Here's how the part is built. I have some questions about the finished solid (model axes, mm). Face numbers are marked on the shaded views. A direction names the side the tool comes from. Coordinates: 2 decimals unless noted, no trailing zeros. Order: outer loops, then holes, each group sorted by start corner. A loop starts at its lowest first (then second) coordinate and runs counter-clockwise, first axis right, second up.
Autodesk Inventor part; units mm, degrees
ref_plane "YZ Plane" through (0, 0, 0) normal (1, 0, 0) x (0, 1, 0)
ref_plane "XZ Plane" through (0, 0, 0) normal (0, 1, 0) x (-1, 0, 0)
ref_plane "XY Plane" through (0, 0, 0) normal (0, 0, 1) x (1, 0, 0)
sketch "Sketch1" plane through (0, 0, 0) normal (0, 0, 1) x (1, 0, 0)
  circle A0 centre (0, 0) radius 5
  dimension "d0" = 10
extrude "Extrusion1" add sketch "Sketch1" along normal blind 3
sketch "Sketch2" plane through (0, 0, 3) normal (0, 0, 1) x (1, 0, 0)
  circle A0 centre (0, 0) radius 5
  line L0 (-5.1933, 1) -> (5.1933, 1)
  line L1 (5.1933, 1) -> (5.1933, -1)
  line L2 (5.1933, -1) -> (-5.1933, -1)
  line L3 (-5.1933, -1) -> (-5.1933, 1)
  line L4 (-5.1933, 1) -> (5.1933, -1) construction
  line L5 (5.1933, 1) -> (-5.1933, -1) construction
  point P0 (-4.899, -1)
  point P1 (4.899, -1)
  point P2 (4.899, 1)
  point P3 (-4.899, 1)
  dimension "d3" = 2
  dimension "d4" = 79.101
extrude "Extrusion2" cut sketch "Sketch2" against normal blind 1 contours A0 L2 L0
fillet "Fillet1" radius 1 2 edges at (0, 5, 3) (0, -5, 3)
sketch "Sketch3" plane through (0, 0, 0) normal (0, 0, -1) x (-1, 0, 0)
  circle A0 centre (0, 0) radius 5
  circle A1 centre (0, 0) radius 3.25
  dimension "d8" = 6.5
extrude "Extrusion3" add sketch "Sketch3" along normal blind 16 contours A1
sketch "Sketch4" plane through (0, 0, -16) normal (0, 0, -1) x (-1, 0, 0)
  circle A0 centre (0, 0) radius 3.25
hole "Hole1" at (0, 0, -16) direction (0, 0, 1) diameter 3.242 depth 8 tip angle 118
properties part number "17B - Crosshead Pin2" material "Steel AISI 1020 107 HR"
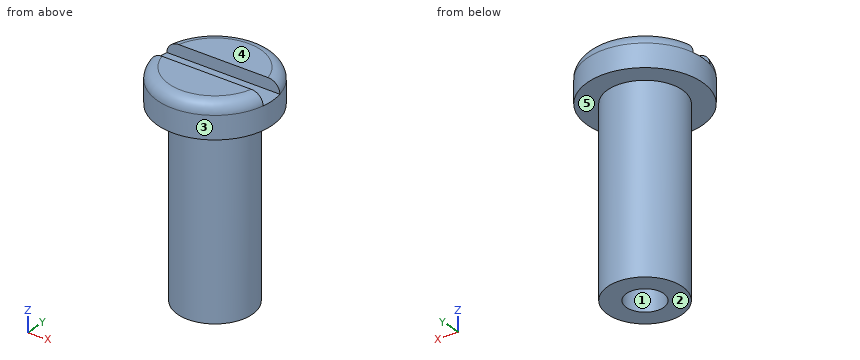
Q1. If we section it at C-C on z = -4: Write out the boundary of the cut face in (x, y), then the cut area to 3 significant figures.
Q2. For the marked faces 4 and 5, which set-ups out of +Z, -Z, +X, -X, +Y, -Y let a thin tool reach every point of the face, with its end or its side?
Q3. If we section it at A-A on z = -11: Write out the boundary of the cut face in (x, y).
Q4. I need wall thicknesses on L1, parallel to Y at x = 0, z = -12; L2, parallel to Z at x = -2, y = -0.5; L3, parallel to Z at x = -3, y = 2.25. Which ranges of each line are inside material? Lowest first, please.
Q5. We'd pull the mould along Y, two halves only. Please class the marked faces 1, 2 and 3: pulls with the +Y half, pulls with the -Y half, needs draft (parallel to the pull), parting line crosses it, or undercut.
Q6. If we section it at B-B on z = 0.25: Write out the boundary of the cut face in (x, y), then the cut area to 3 significant figures.
Q7. Will these pins go through, and if not, where does the flat tip stop? pin 1 (1 mm diameter, centred on x = 0, z = -3.5, fed in from -Y); pin 2 (1 mm diameter, centred on y = 2.5, z = -2, fed in from -X); pin 3 (3 mm diameter, centred on x = -3.5, z = 0, fed in from +Y).
Reply:
1. outline: circle Ø6.5 at (0, 0)
1. area: 33.2 mm2
2. face 4: +Z, +X, -X, +Y, -Y
2. face 5: -Z
3. outline: circle Ø6.5 at (0, 0); hole circle Ø3.24 at (0, 0)
4. L1: y = -3.25 to -1.62, 1.62 to 3.25
4. L2: z = -16 to 2
4. L3: z = 0 to 3
5. face 1: undercut
5. face 2: needs draft
5. face 3: parting line crosses it
6. outline: circle Ø10 at (0, 0)
6. area: 78.5 mm2
7. pin 1: stops at y = -3.25
7. pin 2: stops at x = -2.56
7. pin 3: stops at y = 4.58
